Answer from the drawing. Dimensions are ordinates in mm from the lowest x, y and z of the part. Coordinates: 2 decimals unless noted, no trailing zeros. Order: outer loops, then holes, each group sorted by start corner. A loop starts at its lowest first (then second) coordinate and runs counter-clockwise, first axis right, second up. Notation, with made-up numbers: (36, 68) - (74, 68) arc R9 ccw to (74, 78) - close; hole circle Ø7 at (-39, 57). An arc over 180 degrees is marked (long way). Use a Markdown table: item, result. Add a question column.
Item 1: The part is cut by section C-C, the plane z = 8.5. Give the vertices of the cut face in (x, y).
Item 2: The part is cut by section A-A, the plane y = 27.5. Give the vertices of the cut face in (x, z).
Item 3: Flat-ended cylindrical pins translate along their axes: P1, Ø1.9, axis at x = 22.5, y = 27.5, coming from the -Z side; P2, Ø2, axis at x = 8, y = 26.5, coming from the +Z side. Find the tip coordinate at first contact, or state that the pin passes through.
Item 4: The part is cut by section B-B, the plane x = 7.5. Give the vertices of the cut face in (y, z), then the cut area to 3 significant figures.
Item 5: Find the intervals of material crossed by line 1 along X through (y, z) = (14.5, 8.5); line 2 along Y through (x, z) = (7.5, 8.95); line 3 along Y through (x, z) = (7.5, 2), in increasing order.
Item 6: The part is cut by section D-D, the plane z = 3. Give the vertices of the cut face in (x, y).
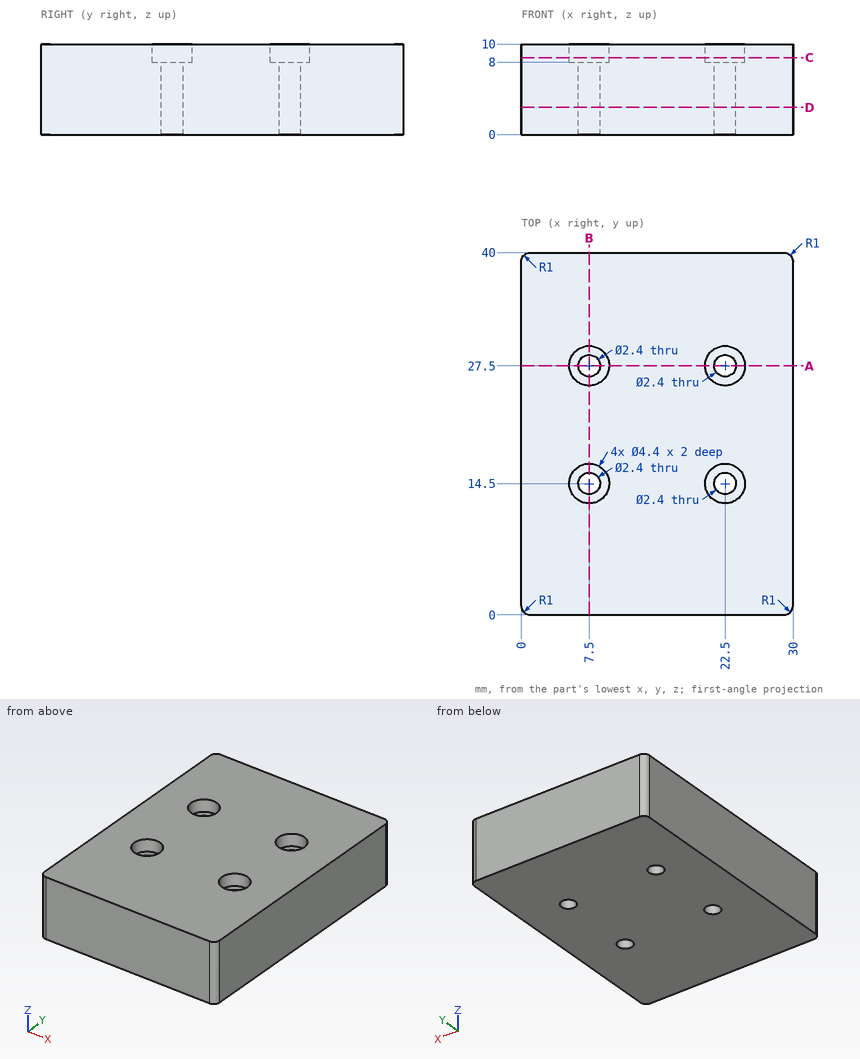
Solution:
| question | item | result |
|---|---|---|
| 1 | outline | (0, 1) arc R1 ccw to (1, 0) - (29, 0) arc R1 ccw to (30, 1) - (30, 39) arc R1 ccw to (29, 40) - (1, 40) arc R1 ccw to (0, 39) - close; hole circle Ø4.4 at (7.5, 14.5); hole circle Ø4.4 at (7.5, 27.5); hole circle Ø4.4 at (22.5, 14.5); hole circle Ø4.4 at (22.5, 27.5) |
| 2 | outline | (0, 0) - (6.3, 0) - (6.3, 8) - (5.3, 8) - (5.3, 10) - (0, 10) - close; (8.7, 0) - (21.3, 0) - (21.3, 8) - (20.3, 8) - (20.3, 10) - (9.7, 10) - (9.7, 8) - (8.7, 8) - close; (23.7, 0) - (30, 0) - (30, 10) - (24.7, 10) - (24.7, 8) - (23.7, 8) - close |
| 3 | P1 | passes through |
| 3 | P2 | stops at z = 8 |
| 4 | outline | (0, 0) - (13.3, 0) - (13.3, 8) - (12.3, 8) - (12.3, 10) - (0, 10) - close; (15.7, 0) - (26.3, 0) - (26.3, 8) - (25.3, 8) - (25.3, 10) - (16.7, 10) - (16.7, 8) - (15.7, 8) - close; (28.7, 0) - (40, 0) - (40, 10) - (29.7, 10) - (29.7, 8) - (28.7, 8) - close |
| 4 | area | 344 mm2 |
| 5 | line 1 | x = 0 to 5.3, 9.7 to 20.3, 24.7 to 30 |
| 5 | line 2 | y = 0 to 12.3, 16.7 to 25.3, 29.7 to 40 |
| 5 | line 3 | y = 0 to 13.3, 15.7 to 26.3, 28.7 to 40 |
| 6 | outline | (0, 1) arc R1 ccw to (1, 0) - (29, 0) arc R1 ccw to (30, 1) - (30, 39) arc R1 ccw to (29, 40) - (1, 40) arc R1 ccw to (0, 39) - close; hole circle Ø2.4 at (7.5, 14.5); hole circle Ø2.4 at (7.5, 27.5); hole circle Ø2.4 at (22.5, 14.5); hole circle Ø2.4 at (22.5, 27.5) |
